Geometry: final body of the model. Coordinates: model frame, mm. Face numbers are marked on the shaded views. A direction names the side the tool comes from. Give positions to 0.01 mm unless a question says otherwise; leave off trailing zeros. Write each loop counter-clockwise with the first axis right and the second up, starting at its lowest first coordinate (ties: lowest second). Pieces come first, ordered by that corner, then holes. Notation, with made-up numbers: (6.25, 63.25) -> (16.25, 63.25) arc R17 ccw to (16.25, 94.25) -> close; hole circle Ø9 at (26.5, 4.25). An arc over 180 degrees is marked (long way). Answer in a Markdown table with one row per item. Add a question column.
Item 1: Section query D-D on z = 23. Output: boundary loops of the cut face in (x, y), plus the area to 3 significant figures.
Item 2: Section query B-B on z = 13. Output: boundary loops of the cut face in (x, y).
Item 3: First-contact query: P1, Ø4, axis at x = -15.5, y = 42.97, coming from the +Z side; P2, Ø3, axis at x = 15.5, y = 73.97, coming from the +Z side; P3, Ø12, axis at x = 15.5, y = 52.5, coming from the -Z side; P4, Ø6, axis at x = -15, z = 15, coming from the +Y side. Flat tips, straight axial feed; report the tip coordinate or a pass-through.
Item 4: Material intervals for probe 1 along X at (y, z) = (24.5, 15); probe 2 along Y at (x, z) = (15.5, 7.55); probe 3 along Y at (x, z) = (0, 5), sorted ascending. Write a range as from..to.
Item 5: Draft query along Y for the marked faces 1, 2 and 3. Return one class per face: +Y half, -Y half, draft (parallel to the pull), parting line (faces both ways), or undercut.
Item 6: Section query C-C on y = 71.5. Output: boundary loops of the cut face in (x, z).
Item 7: Section query A-A on x = -2. Output: boundary loops of the cut face in (y, z), plus the area to 3 significant figures.
Item 8: Access query for the marked faces 4, 5 and 6. Directions: +Z, -Z, +X, -X, +Y, -Y. A direction counts if a zero-diameter tool reaches every point of the face in a straight line with its end or side. Return the directions, or none.
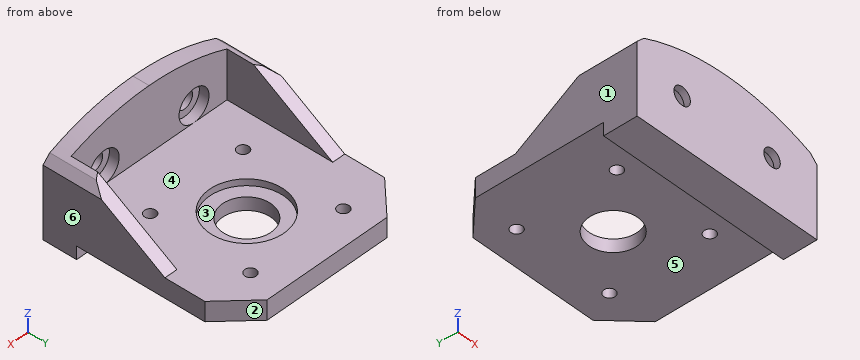
```python
from build123d import *

# Parameters (mm, degrees)
SKETCH1_W                = 120
SKETCH1_H                = 30
BOSS_EXTRUDE1_DEPTH      = 100
SKETCH3_OUTSIDE_W        = 153.812
SKETCH3_OUTSIDE_H        = 133.812
CUT_EXTRUDE2_DEPTH       = 121.415945788
CUT_EXTRUDE3_START       = -30
CUT_EXTRUDE3_DEPTH       = 30
SKETCH5_W                = 67.698745078
SKETCH5_H                = 100.8
CUT_EXTRUDE4_DEPTH       = 20
RIB1_REACH               = 122.416
SKETCH6_WALL_W           = 281.143052644
SKETCH6_WALL_H           = 4
RIB6_REACH               = 122.416
SKETCH7_WALL_W           = 281.143052644
SKETCH7_WALL_H           = 4
CUT_EXTRUDE5_DEPTH       = 84.326168543
CUT_EXTRUDE5_DEPTH_BACK  = 84.326168543
SKETCH9_R                = 2.75
SKETCH10_R               = 5
CUT_EXTRUDE6_DEPTH       = 3
CHAMFER1_SIZE            = 8
CUT_EXTRUDE7_START       = -14.352520936
CUT_EXTRUDE7_DEPTH       = 14.352520936
SKETCH13_W               = 60
SKETCH13_H               = 40
BOSS_EXTRUDE2_DEPTH      = 10
CUT_EXTRUDE8_DEPTH       = 108.204960324
CUT_EXTRUDE8_DEPTH_BACK  = 108.204960324
SKETCH12_R               = 1.75
SKETCH12_R_2             = 7.5
CHAMFER2_SIZE            = 10
SKETCH14_R               = 11.5
CUT_EXTRUDE9_DEPTH       = 1
BOSS_EXTRUDE3_START      = 1
SKETCH16_W               = 42.5
SKETCH16_H               = 42.5
SKETCH16_R               = 1.75
SKETCH16_R_2             = 11.5
BOSS_EXTRUDE3_DEPTH      = 1
SKETCH17_W               = 48.072912132
SKETCH17_H               = 52.974055018
BOSS_EXTRUDE4_DEPTH      = 10
SKETCH17_2_W             = 48.072912132
SKETCH17_2_H             = 52.974055018
CUT_EXTRUDE10_DEPTH      = 108.204960324
CUT_EXTRUDE11_DEPTH      = 108.204960324
CUT_EXTRUDE11_DEPTH_BACK = 108.204960324
SKETCH18_R               = 7.5
SKETCH18_R_2             = 1.75
SKETCH19_R               = 11.5
CUT_EXTRUDE12_DEPTH      = 2
CUT_EXTRUDE13_DEPTH      = 108.204960324
CUT_EXTRUDE13_DEPTH_BACK = 108.204960324
SKETCH20_W               = 88.74197012
SKETCH20_H               = 29.925009901
CHAMFER3_SIZE            = 10
SKETCH22_W               = 69.690835078
SKETCH22_H               = 49.62
CUT_EXTRUDE14_DEPTH      = 4


# Read off the part's stored shape, not the designer's step: Cut-Extrude3, Cut-Extrude7
with BuildPart() as part:
    # Sketch1 → Boss-Extrude1 (new body)
    with BuildSketch(Plane(origin=(0, 0, 0), x_dir=(1, 0, 0), z_dir=(0, 1, 0))):
        with Locations((0, -15)):
            Rectangle(SKETCH1_W, SKETCH1_H)
    extrude(amount=BOSS_EXTRUDE1_DEPTH)

    # Sketch3 outside → Cut-Extrude2 (cut, through all)
    with BuildSketch(Plane.XY.offset(30)):
        with Locations((0, 50)):
            Rectangle(SKETCH3_OUTSIDE_W, SKETCH3_OUTSIDE_H)
        with BuildLine():
            Line((-45, 23.283541889), (45, 23.283541889))
            Line((45, 23.283541889), (19.804596008, 86.568297014))
            ThreePointArc((19.804596008, 86.568297014), (0, 100), (-19.804596008, 86.568297014))
            Line((-19.804596008, 86.568297014), (-45, 23.283541889))
        make_face(mode=Mode.SUBTRACT)
    extrude(amount=-CUT_EXTRUDE2_DEPTH, mode=Mode.SUBTRACT)

    # Cut-Extrude3 outline → Cut-Extrude3 (cut)
    with BuildSketch(Plane.XY.offset(30).offset(CUT_EXTRUDE3_START)):
        Polygon((30, 60.95991045), (30, 23.283541889), (45, 23.283541889), align=None)
        Polygon((-30, 23.283541889), (-30, 60.95991045), (-45, 23.283541889), align=None)
    extrude(amount=CUT_EXTRUDE3_DEPTH, mode=Mode.SUBTRACT)

    # Sketch5 → Cut-Extrude4 (cut)
    with BuildSketch(Plane.XY.offset(30)):
        with Locations((0, 78.683541889)):
            Rectangle(SKETCH5_W, SKETCH5_H)
    extrude(amount=-CUT_EXTRUDE4_DEPTH, mode=Mode.SUBTRACT)

    # Sketch6 wall → Rib1 (add, up to next)
    with BuildSketch(Plane(origin=(-30, 44.62172617, 20), x_dir=(0, -0.852920340981, 0.522041082618), z_dir=(0, 0.522041082618, 0.852920340981)), mode=Mode.PRIVATE) as rib1_sk1:
        with Locations((0, 2)):
            Rectangle(SKETCH6_WALL_W, SKETCH6_WALL_H)
    rib1_tool1 = extrude(rib1_sk1.sketch, amount=-RIB1_REACH, mode=Mode.PRIVATE) - part.part
    add(rib1_tool1.solids().sort_by_distance((-30, 44.62172617, 20))[0])

    # Sketch7 wall → Rib6 (add, up to next)
    with BuildSketch(Plane(origin=(30, 44.62172617, 20), x_dir=(0, -0.852920340981, 0.522041082618), z_dir=(0, -0.522041082618, -0.852920340981)), mode=Mode.PRIVATE) as rib6_sk1:
        with Locations((0, 2)):
            Rectangle(SKETCH7_WALL_W, SKETCH7_WALL_H)
    rib6_tool1 = extrude(rib6_sk1.sketch, amount=RIB6_REACH, mode=Mode.PRIVATE) - part.part
    add(rib6_tool1.solids().sort_by_distance((30, 44.62172617, 20))[0])

    # Sketch9 → Cut-Extrude5 (cut, two sides: drawn at the far end of the back side and taken through both)
    with BuildSketch(Plane(origin=(0, 28.283541889, 0), x_dir=(1, 0, 0), z_dir=(0, 1, 0)).offset(-CUT_EXTRUDE5_DEPTH_BACK)):
        with Locations(Location((-15, -15, 0), (0, 0, 270))):
            Circle(SKETCH9_R)
        with Locations(Location((15, -15, 0), (0, 0, 270))):
            Circle(SKETCH9_R)
    extrude(amount=CUT_EXTRUDE5_DEPTH + CUT_EXTRUDE5_DEPTH_BACK, mode=Mode.SUBTRACT)

    # Sketch10 → Cut-Extrude6 (cut)
    with BuildSketch(Plane(origin=(0, 28.283541889, 0), x_dir=(1, 0, 0), z_dir=(0, 1, 0))):
        with Locations((-15, -15)):
            Circle(SKETCH10_R)
        with Locations((15, -15)):
            Circle(SKETCH10_R)
    extrude(amount=-CUT_EXTRUDE6_DEPTH, mode=Mode.SUBTRACT)

    # Chamfer1
    # the kernel refuses this chamfer: 8 mm, written as the material it takes off along each edge
    with BuildSketch(Plane(origin=(-30, 2.710077985, 30), x_dir=(-0.027495876610586535, 0, -0.9996219169112968), z_dir=(0, 1, 0))) as chamfer1_piece_1:
        Polygon((CHAMFER1_SIZE * 0.999621916911, -CHAMFER1_SIZE * 0.0274958766106), (-CHAMFER1_SIZE * 0.0274958766106, -CHAMFER1_SIZE * 0.999621916911), (0, 0), align=None)
    extrude(amount=46.146927807, mode=Mode.SUBTRACT)
    with BuildSketch(Plane(origin=(30, 48.857005793, 30), x_dir=(-0.9996219169112968, 0, 0.027495876610586487), z_dir=(0, -1, 0))) as chamfer1_piece_2:
        Polygon((CHAMFER1_SIZE * 0.999621916911, CHAMFER1_SIZE * 0.0274958766106), (-CHAMFER1_SIZE * 0.0274958766106, CHAMFER1_SIZE * 0.999621916911), (0, 0), align=None)
    extrude(amount=46.146927807, mode=Mode.SUBTRACT)

    # Cut-Extrude7 outline → Cut-Extrude7 (cut)
    with BuildSketch(Plane.XZ.offset(-23.283541889).offset(CUT_EXTRUDE7_START)):
        with BuildLine():
            ThreePointArc((-27.724333118, 24.275666882), (-14.154563191, 28.553981218), (0, 30))
            Line((0, 30), (-22, 30))
            Line((-22, 30), (-27.724333118, 24.275666882))
        make_face()
        with BuildLine():
            ThreePointArc((0, 30), (14.154563191, 28.553981218), (27.724333118, 24.275666882))
            Line((27.724333118, 24.275666882), (22, 30))
            Line((22, 30), (0, 30))
        make_face()
    extrude(amount=CUT_EXTRUDE7_DEPTH, mode=Mode.SUBTRACT)

    # Sketch13 → Boss-Extrude2 (add)
    with BuildSketch(Plane(origin=(0, 0, 0), x_dir=(-1, 0, 0), z_dir=(0, 0, -1))):
        with Locations((0, 80.95991045)):
            Rectangle(SKETCH13_W, SKETCH13_H)
    extrude(amount=-BOSS_EXTRUDE2_DEPTH)

    # Sketch12 → Cut-Extrude8 (cut, two sides: drawn at the far end of the back side and taken through both)
    with BuildSketch(Plane.XY.offset(10).offset(-CUT_EXTRUDE8_DEPTH_BACK)):
        with Locations((-15.5, 84.083541889)):
            Circle(SKETCH12_R)
        with Locations((15.5, 84.083541889)):
            Circle(SKETCH12_R)
        with Locations((-15.5, 53.083541889)):
            Circle(SKETCH12_R)
        with Locations((15.5, 53.083541889)):
            Circle(SKETCH12_R)
        with Locations((0, 68.583541889)):
            Circle(SKETCH12_R_2)
    extrude(amount=CUT_EXTRUDE8_DEPTH + CUT_EXTRUDE8_DEPTH_BACK, mode=Mode.SUBTRACT)

    # Chamfer2
    chamfer2_edges = [part.edges().sort_by_distance(p)[0] for p in [
        (-30, 100.95991045, 5),
        (30, 100.95991045, 5),
    ]]
    chamfer(chamfer2_edges, length=CHAMFER2_SIZE)

    # Sketch14 → Cut-Extrude9 (cut)
    with BuildSketch(Plane.XY.offset(10)):
        with Locations((0, 68.583541889)):
            Circle(SKETCH14_R)
    extrude(amount=-CUT_EXTRUDE9_DEPTH, mode=Mode.SUBTRACT)

    # Sketch16 → Boss-Extrude3 (add)
    with BuildSketch(Plane.XY.offset(10).offset(BOSS_EXTRUDE3_START)):
        with Locations((0, 68.583541889)):
            Rectangle(SKETCH16_W, SKETCH16_H)
        with Locations((-15.5, 84.083541889)):
            Circle(SKETCH16_R, mode=Mode.SUBTRACT)
        with Locations((15.5, 84.083541889)):
            Circle(SKETCH16_R, mode=Mode.SUBTRACT)
        with Locations((15.5, 53.083541889)):
            Circle(SKETCH16_R, mode=Mode.SUBTRACT)
        with Locations((-15.5, 53.083541889)):
            Circle(SKETCH16_R, mode=Mode.SUBTRACT)
        with Locations((0, 68.583541889)):
            Circle(SKETCH16_R_2, mode=Mode.SUBTRACT)
    extrude(amount=-BOSS_EXTRUDE3_DEPTH)

    # Sketch17 → Boss-Extrude4 (add)
    with BuildSketch(Plane.XY.offset(10)):
        with Locations((0, 67.231428327)):
            Rectangle(SKETCH17_W, SKETCH17_H)
    extrude(amount=-BOSS_EXTRUDE4_DEPTH)

    # Sketch17<2> → Cut-Extrude10 (cut, through all)
    with BuildSketch(Plane.XY.offset(10)):
        with Locations((0, 67.231428327)):
            Rectangle(SKETCH17_2_W, SKETCH17_2_H)
    extrude(amount=CUT_EXTRUDE10_DEPTH, mode=Mode.SUBTRACT)

    # Sketch18 → Cut-Extrude11 (cut, two sides: drawn at the far end of the back side and taken through both)
    with BuildSketch(Plane.XY.offset(10).offset(-CUT_EXTRUDE11_DEPTH_BACK)):
        with Locations((0, 58.473541889)):
            Circle(SKETCH18_R)
        with Locations((-15.5, 73.973541889)):
            Circle(SKETCH18_R_2)
        with Locations((-15.5, 42.973541889)):
            Circle(SKETCH18_R_2)
        with Locations((15.5, 42.973541889)):
            Circle(SKETCH18_R_2)
        with Locations((15.5, 73.973541889)):
            Circle(SKETCH18_R_2)
    extrude(amount=CUT_EXTRUDE11_DEPTH + CUT_EXTRUDE11_DEPTH_BACK, mode=Mode.SUBTRACT)

    # Sketch19 → Cut-Extrude12 (cut)
    with BuildSketch(Plane.XY.offset(10)):
        with Locations((0, 58.473541889)):
            Circle(SKETCH19_R)
    extrude(amount=-CUT_EXTRUDE12_DEPTH, mode=Mode.SUBTRACT)

    # Sketch20 → Cut-Extrude13 (cut, two sides: drawn at the far end of the back side and taken through both)
    with BuildSketch(Plane.XY.offset(10).offset(-CUT_EXTRUDE13_DEPTH_BACK)):
        with Locations((2.815550168, 98.246046839)):
            Rectangle(SKETCH20_W, SKETCH20_H)
    extrude(amount=CUT_EXTRUDE13_DEPTH + CUT_EXTRUDE13_DEPTH_BACK, mode=Mode.SUBTRACT)

    # Chamfer3
    chamfer3_edges = [part.edges().sort_by_distance(p)[0] for p in [
        (30, 83.283541889, 5),
        (-30, 83.283541889, 5),
    ]]
    chamfer(chamfer3_edges, length=CHAMFER3_SIZE)

    # Sketch22 → Cut-Extrude14 (cut)
    with BuildSketch(Plane(origin=(0, 0, 0), x_dir=(-1, 0, 0), z_dir=(0, 0, -1))):
        with Locations((0, 58.473541889)):
            Rectangle(SKETCH22_W, SKETCH22_H)
    extrude(amount=-CUT_EXTRUDE14_DEPTH, mode=Mode.SUBTRACT)


solid = part.part
```
Findings below:
| question | item | result |
|---|---|---|
| 1 | outline | (-29, 23.28) -> (29, 23.28) -> (29, 39.72) -> (26, 39.72) -> (26, 28.28) -> (-26, 28.28) -> (-26, 39.72) -> (-29, 39.72) -> close |
| 1 | area | 359 mm^2 |
| 2 | outline | (-30, 23.28) -> (-16.89, 23.28) -> (-16.89, 25.28) -> (-19.58, 25.28) -> (-19.58, 28.28) -> (-26, 28.28) -> (-26, 56.06) -> (-30, 56.06) -> close; (-13.11, 23.28) -> (13.11, 23.28) -> (13.11, 25.28) -> (10.42, 25.28) -> (10.42, 28.28) -> (-10.42, 28.28) -> (-10.42, 25.28) -> (-13.11, 25.28) -> close; (16.89, 23.28) -> (30, 23.28) -> (30, 56.06) -> (26, 56.06) -> (26, 28.28) -> (19.58, 28.28) -> (19.58, 25.28) -> (16.89, 25.28) -> close |
| 3 | P1 | stops at z = 10 |
| 3 | P2 | passes through |
| 3 | P3 | stops at z = 4 |
| 3 | P4 | stops at y = 25.28 |
| 4 | probe 1 | x = -30..-17.75, -12.25..12.25, 17.75..30 |
| 4 | probe 2 | y = 23.28..41.22, 44.72..72.22, 75.72..83.28 |
| 4 | probe 3 | y = 23.28..50.97, 65.97..83.28 |
| 5 | face 1 | draft |
| 5 | face 2 | +Y half |
| 5 | face 3 | undercut |
| 6 | outline | (-30, 4) -> (30, 4) -> (30, 10) -> (-30, 10) -> close |
| 7 | outline | (23.28, 0) -> (33.66, 0) -> (33.66, 4) -> (51.25, 4) -> (51.25, 8) -> (47.15, 8) -> (47.15, 10) -> (28.28, 10) -> (28.28, 29.97) -> (23.28, 29.97) -> close; (65.7, 4) -> (83.28, 4) -> (83.28, 10) -> (69.8, 10) -> (69.8, 8) -> (65.7, 8) -> close |
| 7 | area | 398 mm^2 |
| 8 | face 4 | +Z, +Y |
| 8 | face 5 | -Z, +X, -X, +Y |
| 8 | face 6 | +Z, -Z, +X, +Y, -Y |
